Geometry: see drawing. Coordinates: mm, zero at the bounding-box minimum. A direction names the side the tool comes from. Round coordinates to 2 decimals unless told otherwise and drop trailing zeros. Loops run counter-clockwise (first coordinate to the right, second up) from the corner with the lowest first, then second, coordinate; pieces in that order, holes last. Notation, with made-up numbers: (17.5, 33.5) - (24.5, 33.5) arc R19 ccw to (24.5, 58.5) - close; hole circle Ø7 at (1.25, -17.75). An arc over 180 degrees is marked (long way). Answer in a Markdown table with one row per item. Add a question column.
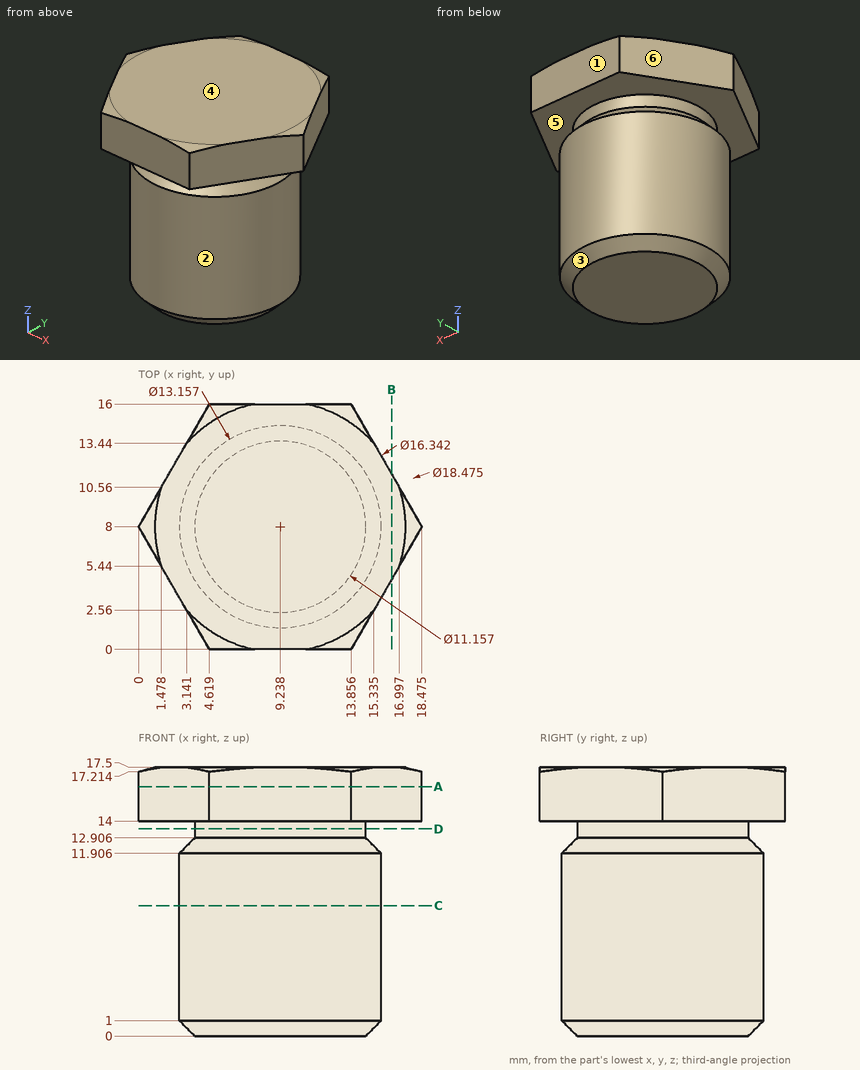
1) Section B-B, the plane x = 16.5. Return the cut outline in (y, z).
2) Pull-direction query (Z, two-part tool) for the marked faces 3, 4, 5 and 6; classes: pulls with the +Z half, pulls with the -Z half, needs draft (parallel to the pull), parting line crosses it, or undercut.
3) Reachability of the marked faces 1 and 2 from +Z, -Z, +X, -X, +Y, -Y: full face, straight path, thin tool, end or side. Return the list, or none.
4) Material intervals for line 1 along Z through (x, y) = (8, 1.75) (1 decimal); line 2 along Z through (x, y) = (3.5, 3); line 3 along X through (y, z) = (5.75, 1.25) (1 decimal), sorted ascending. Write a range as from..to.
5) Section D-D, the plane z = 13.5. Return the cut outline in (x, y).
6) Section C-C, the plane z = 8.5. Return the cut outline in (x, y).
7) Section A-A, the plane z = 16.25. Return the cut outline in (x, y) (1 decimal), and give its area (3 significant figures).
8) Contact query for flat-ended pins moving along their axis: pin 1 Ø4 at (x, z) = (15.5, 4.5) entering from +Y; pin 2 Ø1.5 at (y, z) = (3, 14.5) entering from +X; pin 3 Ø6 at (y, z) = (2, 10) entering from +X. Output: stop coordinate, or through.
Evaluation:
| question | item | result |
|---|---|---|
| 1 | outline | (4.58, 14) - (11.42, 14) - (11.42, 17.5) - (4.58, 17.5) - close |
| 2 | face 3 | pulls with the -Z half |
| 2 | face 4 | pulls with the +Z half |
| 2 | face 5 | undercut |
| 2 | face 6 | needs draft |
| 3 | face 1 | +Z, -Z, +X, -X, +Y |
| 3 | face 2 | -Z |
| 4 | line 1 | z = 0.8..12.1, 14..17.5 |
| 4 | line 2 | z = 14..17.5 |
| 4 | line 3 | x = 3.1..15.4 |
| 5 | outline | circle Ø11.16 at (9.24, 8) |
| 6 | outline | circle Ø13.16 at (9.24, 8) |
| 7 | outline | (0, 8) - (4.6, 0) - (13.9, 0) - (18.5, 8) - (13.9, 16) - (4.6, 16) - close |
| 7 | area | 222 mm² |
| 8 | pin 1 | stops at y = 13.01 |
| 8 | pin 2 | stops at x = 16.02 |
| 8 | pin 3 | stops at x = 15.09 |
